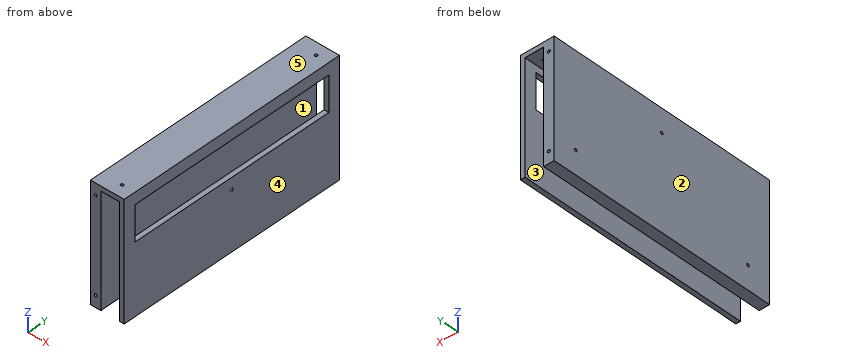
```python
from build123d import *

# Parameters (mm, degrees)
SKETCH1_W                 = 29
SKETCH1_H                 = 100
BOSS_EXTRUDE1_DEPTH       = 200
SKETCH2_W                 = 16
SKETCH2_H                 = 96
CUT_EXTRUDE1_DEPTH        = 207.664583323
SKETCH3_W                 = 30
SKETCH3_H                 = 180
CUT_EXTRUDE2_DEPTH        = 4
M2_CLEARANCE_HOLE1_D      = 2.4
M2_CLEARANCE_HOLE1_DEPTH  = 11.2
M2_CLEARANCE_HOLE1_TIP    = 0.721032743
M2_CLEARANCE_HOLE2_D      = 2.4
M2_CLEARANCE_HOLE2_DEPTH  = 11.2
M2_CLEARANCE_HOLE2_TIP    = 0.721032743
M2_CLEARANCE_HOLE3_REACH  = 210.185
M2_CLEARANCE_HOLE3_BORE_R = 1.2
M2_CLEARANCE_HOLE4_REACH  = 210.185
M2_CLEARANCE_HOLE4_BORE_R = 1.2
M2_CLEARANCE_HOLE5_D      = 2.4


with BuildPart() as part:
    # Sketch1 → Boss-Extrude1 (new body)
    with BuildSketch(Plane(origin=(0, 0, 0), x_dir=(1, 0, 0), z_dir=(0, 1, 0))):
        Rectangle(SKETCH1_W, SKETCH1_H)
    extrude(amount=BOSS_EXTRUDE1_DEPTH)

    # Sketch2 → Cut-Extrude1 (cut, through all)
    with BuildSketch(Plane(origin=(0, 200, 0), x_dir=(1, 0, 0), z_dir=(0, 1, 0))):
        with Locations((2.5, 2)):
            Rectangle(SKETCH2_W, SKETCH2_H)
    extrude(amount=-CUT_EXTRUDE1_DEPTH, mode=Mode.SUBTRACT)

    # Sketch3 → Cut-Extrude2 (cut)
    with BuildSketch(Plane(origin=(14.5, 0, 0), x_dir=(0, 0, -1), z_dir=(1, 0, 0))):
        with Locations((-25, 100)):
            Rectangle(SKETCH3_W, SKETCH3_H)
    extrude(amount=-CUT_EXTRUDE2_DEPTH, mode=Mode.SUBTRACT)

    # M2 Clearance Hole1
    with Locations(Plane(origin=(0, 200, 0), x_dir=(1, 0, 0), z_dir=(0, 1, 0))):
        with Locations((-10, 40), (-10, -40)):
            Hole(M2_CLEARANCE_HOLE1_D / 2, depth=M2_CLEARANCE_HOLE1_DEPTH)
            with Locations((0, 0, -(M2_CLEARANCE_HOLE1_DEPTH + M2_CLEARANCE_HOLE1_TIP / 2))):  # 118° drill point
                Cone(0, M2_CLEARANCE_HOLE1_D / 2, M2_CLEARANCE_HOLE1_TIP, mode=Mode.SUBTRACT)

    # M2 Clearance Hole2
    with Locations(Plane(origin=(0, 0, 0), x_dir=(-1, 0, 0), z_dir=(0, -1, 0))):
        with Locations((10, 40), (10, -40)):
            Hole(M2_CLEARANCE_HOLE2_D / 2, depth=M2_CLEARANCE_HOLE2_DEPTH)
            with Locations((0, 0, -(M2_CLEARANCE_HOLE2_DEPTH + M2_CLEARANCE_HOLE2_TIP / 2))):  # 118° drill point
                Cone(0, M2_CLEARANCE_HOLE2_D / 2, M2_CLEARANCE_HOLE2_TIP, mode=Mode.SUBTRACT)

    # M2 Clearance Hole3 bore → M2 Clearance Hole3 (cut, up to next)
    with BuildSketch(Plane.ZY.offset(14.5), mode=Mode.PRIVATE) as m2_clearance_hole3_sk1:
        with Locations((-30, 180)):
            Circle(M2_CLEARANCE_HOLE3_BORE_R)
    m2_clearance_hole3_tool1 = extrude(m2_clearance_hole3_sk1.sketch, amount=-M2_CLEARANCE_HOLE3_REACH, mode=Mode.PRIVATE) & part.part
    # M2 Clearance Hole3 bore → M2 Clearance Hole3 (cut, up to next)
    with BuildSketch(Plane.ZY.offset(14.5), mode=Mode.PRIVATE) as m2_clearance_hole3_sk2:
        with Locations((-30, 20)):
            Circle(M2_CLEARANCE_HOLE3_BORE_R)
    m2_clearance_hole3_tool2 = extrude(m2_clearance_hole3_sk2.sketch, amount=-M2_CLEARANCE_HOLE3_REACH, mode=Mode.PRIVATE) & part.part
    # M2 Clearance Hole3 bore → M2 Clearance Hole3 (cut, up to next)
    with BuildSketch(Plane.ZY.offset(14.5), mode=Mode.PRIVATE) as m2_clearance_hole3_sk3:
        with Locations((30, 100)):
            Circle(M2_CLEARANCE_HOLE3_BORE_R)
    m2_clearance_hole3_tool3 = extrude(m2_clearance_hole3_sk3.sketch, amount=-M2_CLEARANCE_HOLE3_REACH, mode=Mode.PRIVATE) & part.part
    add(m2_clearance_hole3_tool1.solids().sort_by_distance((-14.5, 180, -30))[0], mode=Mode.SUBTRACT)
    add(m2_clearance_hole3_tool2.solids().sort_by_distance((-14.5, 20, -30))[0], mode=Mode.SUBTRACT)
    add(m2_clearance_hole3_tool3.solids().sort_by_distance((-14.5, 100, 30))[0], mode=Mode.SUBTRACT)

    # M2 Clearance Hole4 bore → M2 Clearance Hole4 (cut, up to next)
    with BuildSketch(Plane(origin=(14.5, 0, 0), x_dir=(0, 0, -1), z_dir=(1, 0, 0)), mode=Mode.PRIVATE) as m2_clearance_hole4_sk1:
        with Locations((0, 100)):
            Circle(M2_CLEARANCE_HOLE4_BORE_R)
    m2_clearance_hole4_tool1 = extrude(m2_clearance_hole4_sk1.sketch, amount=-M2_CLEARANCE_HOLE4_REACH, mode=Mode.PRIVATE) & part.part
    add(m2_clearance_hole4_tool1.solids().sort_by_distance((14.5, 100, 0))[0], mode=Mode.SUBTRACT)

    # M2 Clearance Hole5 (through all)
    with Locations(Plane.XY.offset(50)):
        with Locations((3.5, 10), (3.5, 190)):
            Hole(M2_CLEARANCE_HOLE5_D / 2)


solid = part.part
```
Verification items for the finished model (mm, model axes). Face numbers are marked on the shaded views. A direction names the side the tool comes from. Give positions to 0.01 mm unless a question says otherwise; leave off trailing zeros. Order: outer loops, then holes, each group sorted by start corner. A loop starts at its lowest first (then second) coordinate and runs counter-clockwise, first axis right, second up. Notation, with made-up numbers: (28, 78) -> (32, 78) arc R12 cw to (32, 95) -> close; hole circle Ø1 at (-1.75, 45.5). An arc over 180 degrees is marked (long way). Use a Markdown table: item, result.
1) Depth check by flat-ended pin: pin 1 Ø5 at (x, z) = (6, -14.5) entering from -Y; pin 2 Ø2 at (x, z) = (-10, -40) entering from +Y; pin 3 Ø2 at (x, y) = (7.5, 159.5) entering from -Z; pin 4 Ø5 at (y, z) = (88, 14.5) entering from +X. Enter the tip coordinate at first touch or a pass-through.
Results:
| item | result |
|---|---|
| pin 1 | through |
| pin 2 | y = 188.68 |
| pin 3 | z = 46 |
| pin 4 | x = -5.5 |
2) Section check C-C, the plane z = -19. Record the boundary of the cut face in (x, y).
Results:
| item | result |
|---|---|
| outline | (-14.5, 0) -> (-5.5, 0) -> (-5.5, 200) -> (-14.5, 200) -> close; (10.5, 0) -> (14.5, 0) -> (14.5, 200) -> (10.5, 200) -> close |
3) Section check B-B, the plane y = 87.5. Record the boundary of the cut face in (x, z).
Results:
| item | result |
|---|---|
| outline | (-14.5, -50) -> (-5.5, -50) -> (-5.5, 46) -> (10.5, 46) -> (10.5, 40) -> (14.5, 40) -> (14.5, 50) -> (-14.5, 50) -> close; (10.5, -50) -> (14.5, -50) -> (14.5, 10) -> (10.5, 10) -> close |
4) Tool access check on the marked faces 1 and 2. Record the directions out of +Z, -Z, +X, -X, +Y, -Y that give a thin tool (end or side, any length) a straight path to the whole face; none if there is none.
Results:
| item | result |
|---|---|
| face 1 | -Z, +Y, -Y |
| face 2 | +Z, -Z, -X, +Y, -Y |
5) Section check A-A, the plane z = 36. Record the boundary of the cut face in (x, y).
Results:
| item | result |
|---|---|
| outline | (-14.5, 0) -> (-5.5, 0) -> (-5.5, 200) -> (-14.5, 200) -> close; (10.5, 0) -> (14.5, 0) -> (14.5, 10) -> (10.5, 10) -> close; (10.5, 190) -> (14.5, 190) -> (14.5, 200) -> (10.5, 200) -> close |
6) Mould release check, pull along X, two halves, no side actions. Record for the marked faces 3, 4 and 5: pulls with the +X half, pulls with the -X half, needs draft (parallel to the pull), parting line crosses it, or undercut.
Results:
| item | result |
|---|---|
| face 3 | undercut |
| face 4 | pulls with the +X half |
| face 5 | needs draft |
7) Section check D-D, the plane x = -0.5. Record the boundary of the cut face in (y, z), then the cut area to 3 significant figures.
Results:
| item | result |
|---|---|
| outline | (0, 46) -> (200, 46) -> (200, 50) -> (0, 50) -> close |
| area | 800 mm² |
8) Material ranges on probe 1 along Y at (x, z) = (-7.25, -30); probe 2 along X at (y, z) = (196.5, 40); probe 3 along Y at (x, z) = (3.5, 47.75), recorded low to high.
Results:
| item | result |
|---|---|
| probe 1 | 0 to 18.8, 21.2 to 178.8, 181.2 to 200 |
| probe 2 | -14.5 to -11.2, -8.8 to -5.5, 10.5 to 14.5 |
| probe 3 | 0 to 8.8, 11.2 to 188.8, 191.2 to 200 |
